Design review of the part built by this model. Coordinates are the model's own, in mm. A direction names the side the tool comes from. Coordinates: 2 decimals unless noted, no trailing zeros. Order: outer loops, then holes, each group sorted by start corner. A loop starts at its lowest first (then second) coordinate and runs counter-clockwise, first axis right, second up. Notation, with made-up numbers: (17, 49) -> (50, 49) arc R21 cw to (50, 61) -> close; hole circle Ø8 at (48.25, -4.75). An arc over 180 degrees is marked (long way). Use a Markdown table: item, result. Add a question column.
Q1. Add section C-C (z = 2.3). Count the separate pieces of the cut face and the enclosed holes in it, then the cut area to 3 significant figures.
Q2. Machinability: for faces 5 (the face through (-41.784, 61.955, 1.417)), 6 (the face through (-67, 41.275, 1)), 7 (the face through (9, 103.275, 1)), which of the approach directions +Z, -Z, +X, -X, +Y, -Y give a long, thin tool a straight path to every point of the face, cutting with its end or side? Answer none if there is none.
Q3. Add section D-D (x = -5.5). State the section outline as (y, z) points, then the cut area to 3 significant figures.
Q4. Wall thickness on probe 1 along X at (y, z) = (95, 2.1); probe 2 along X at (y, z) = (99, 0.55); probe 3 along X at (y, z) = (79, 1.7): over which ranges is each line inside the solid? List them lowest first.
Q5. Insertion check: pin 1 (1.4 mm diameter, centred on y = -1, z = 0.5, fed in from +X); pin 2 (1.4 mm diameter, centred on x = -67, z = 1, fed in from +Y) (3 decimals). Each pin has a flat end and moves straight along its axis. Give the tip position at first contact, or say it passes through.
Q6. The part is to be moulded in two halves that separate along Y. For faces 1 (the face through (-68, 0, 1)), 2 (the face through (-69.475, 52, 1)), 3 (the face through (-4, 106.069, 1)), 4 (the face through (-65.094, 94, 1)), say which applies: pulls with the +Y half, pulls with the -Y half, needs draft (parallel to the pull), parting line crosses it, or undercut.
Q7. Add section A-A (y = 8). State the section outline as (x, z) points, then the cut area to 3 significant figures.
Q8. Add section B-B (x = 7.5). State the section outline as (y, z) points (1 decimal), then the cut area to 3 significant figures.
from build123d import *

# Parameters (mm, degrees)
BOSS_EXTRUDE1_DEPTH = 2.794
FILLET1_R           = 7.62
SKETCH2_W           = 6.35
SKETCH2_H           = 1.5875
SKETCH2_W_2         = 2.794
SKETCH2_H_2         = 6.35
CUT_EXTRUDE1_DEPTH  = 127.827697441
FILLET2_R           = 6.35


with BuildPart() as part:
    # Sketch1 → Boss-Extrude1 (new body)
    with BuildSketch(Plane.XY):
        Polygon((18.662640042, 103.275), (-0.387359958, 103.275), (-0.387359958, 106.069), (-6.737359958, 106.069), (-6.737359958, 59.782284891), (-44.075359958, 59.782284891), (-44.075359958, 106.069), (-50.425359958, 106.069), (-50.425359958, 103.275), (-69.475359958, 103.275), (-69.475359958, 0), (-66.300359958, 0), (-66.300359958, -2.794), (-59.950359958, -2.794), (-59.950359958, 0), (-14.2875, 0), (-14.2875, -2.794), (-7.9375, -2.794), (-7.9375, 0), (18.662640042, 0), align=None)
    extrude(amount=BOSS_EXTRUDE1_DEPTH)

    # Fillet1
    fillet1_edges = [part.edges().sort_by_distance(p)[0] for p in [
        (-44.075359958, 59.782284891, 1.397),
        (-6.737359958, 59.782284891, 1.397),
    ]]
    fillet(fillet1_edges, radius=FILLET1_R)

    # Sketch2 → Cut-Extrude1 (cut, through all)
    with BuildSketch(Plane.XY.offset(2.794)):
        with Locations((-56.775359958, 99.30625)):
            Rectangle(SKETCH2_W, SKETCH2_H)
        with Locations((5.962640042, 99.30625)):
            Rectangle(SKETCH2_W, SKETCH2_H)
        with Locations((15.678140042, 44.45)):
            Rectangle(SKETCH2_W_2, SKETCH2_H_2)
        with Locations((15.678140042, 93.75)):
            Rectangle(SKETCH2_W_2, SKETCH2_H_2)
        with Locations((-66.490859958, 93.75)):
            Rectangle(SKETCH2_W_2, SKETCH2_H_2)
        with Locations((-66.490859958, 44.45)):
            Rectangle(SKETCH2_W_2, SKETCH2_H_2)
        with Locations((-66.490859958, 9.525)):
            Rectangle(SKETCH2_W_2, SKETCH2_H_2)
    extrude(amount=-CUT_EXTRUDE1_DEPTH, mode=Mode.SUBTRACT)

    # Fillet2
    fillet2_edges = [part.edges().sort_by_distance(p)[0] for p in [
        (18.662640042, 0, 1.397),
    ]]
    fillet(fillet2_edges, radius=FILLET2_R)


solid = part.part
Established:
| question | item | result |
|---|---|---|
| 1 | separate pieces | 1 |
| 1 | enclosed holes | 7 |
| 1 | area | 7,460 mm^2 |
| 2 | face 5 | +Z, -Z, +Y |
| 2 | face 6 | +Z, -Z |
| 2 | face 7 | +Z, -Z, +X, +Y |
| 3 | outline | (0, 0) -> (106.07, 0) -> (106.07, 2.79) -> (0, 2.79) -> close |
| 3 | area | 296 mm^2 |
| 4 | probe 1 | -69.48 to -67.89, -65.09 to -44.08, -6.74 to 14.28, 17.08 to 18.66 |
| 4 | probe 2 | -69.48 to -59.95, -53.6 to -44.08, -6.74 to 2.79, 9.14 to 18.66 |
| 4 | probe 3 | -69.48 to -44.08, -6.74 to 18.66 |
| 5 | pin 1 | x = -7.94 |
| 5 | pin 2 | y = 103.275 |
| 6 | face 1 | pulls with the -Y half |
| 6 | face 2 | needs draft |
| 6 | face 3 | pulls with the +Y half |
| 6 | face 4 | undercut |
| 7 | outline | (-69.48, 0) -> (-67.89, 0) -> (-67.89, 2.79) -> (-69.48, 2.79) -> close; (-65.09, 0) -> (18.66, 0) -> (18.66, 2.79) -> (-65.09, 2.79) -> close |
| 7 | area | 238 mm^2 |
| 8 | outline | (0, 0) -> (98.5, 0) -> (98.5, 2.8) -> (0, 2.8) -> close; (100.1, 0) -> (103.3, 0) -> (103.3, 2.8) -> (100.1, 2.8) -> close |
| 8 | area | 284 mm^2 |
